Print and shaded views of the part. All mm, measured from the part's lowest x, y and z. A direction names the side the tool comes from. Coordinates: 2 decimals unless noted, no trailing zeros. Loops run counter-clockwise (first coordinate to the right, second up) from the corner with the lowest first, then second, coordinate; pieces in that order, holes last. Notation, with made-up numbers: M 35,-22 L 73,-22 A15 ccw 73,-18 Z; hole C -0.75,52.5 d8. An arc over 180 degrees is marked long. One line per question, with ' | ' between items. Start each with the question number.
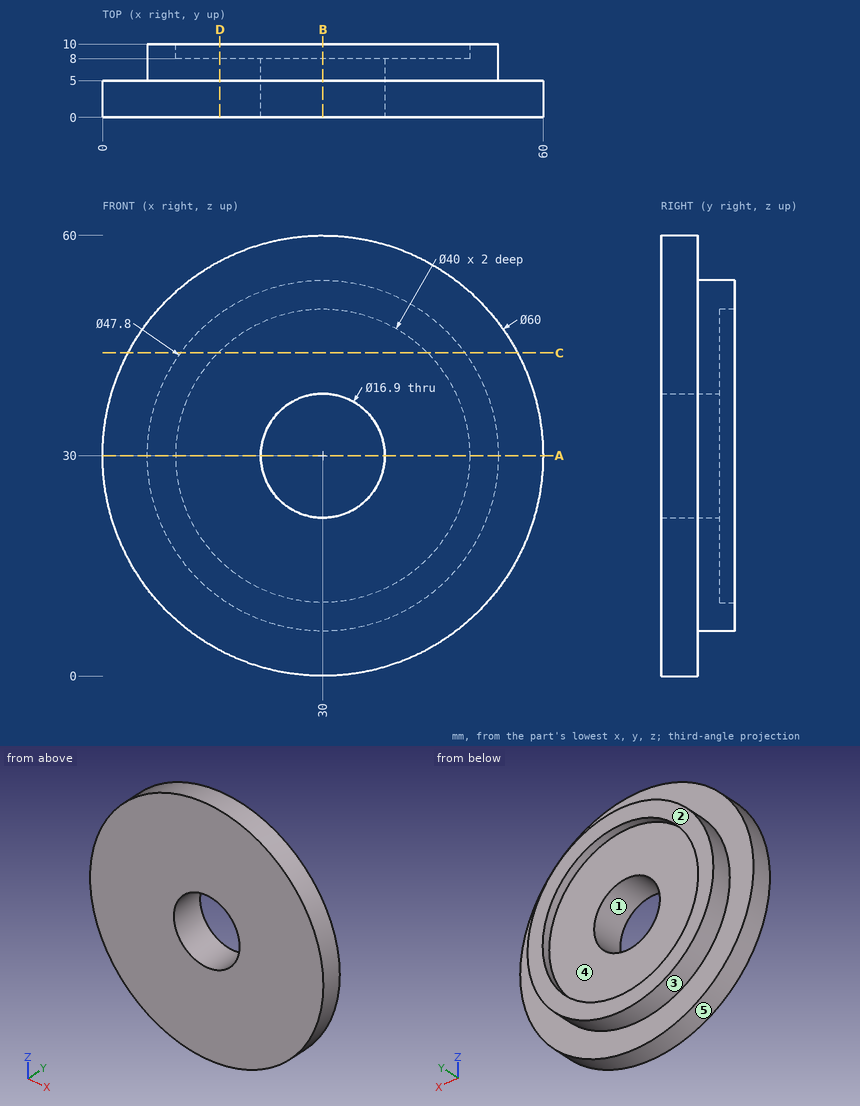
(1) Band-saw the part on B-B on x = 30. Write the cut outline in (y, z).
(2) Band-saw the part on C-C on z = 44. Write the cut outline in (x, y).
(3) Pin check, flat tips, straight feed: P1, Ø2, axis at x = 13, y = 5, coming from the +Z side; P2, Ø6, axis at x = 34.5, y = 2.5, coming from the +Z side; P3, Ø22, axis at x = 30, z = 30, coming from the +Y side. Stop position of each tip, or through.
(4) Drill centre lines: line 1 (X direction, y = 8.85, z = 30); line 2 (X direction, y = 4.5, z = 30). Where is each one in solid material? Low to high. Write a range as [from, to].
(5) Band-saw the part on D-D on x = 16. Write the cut outline in (y, z).
(6) Two-plate mould, pull along Z, no slides. Class the marked faces 1, 2 and 3: pulls with the +Z half, pulls with the -Z half, needs draft (parallel to the pull), parting line crosses it, or undercut.
(7) Band-saw the part on A-A on z = 30. Write the cut outline in (x, y).
(8) 3-axis set-ups, long thin cutter, end or side, ignore diameter. For the marked faces 4 and 5: which of +Z, -Z, +X, -X, +Y, -Y reach the whole face in a straight line?
Computed values:
1) outline: M 0,0 L 5,0 L 5,6.1 L 10,6.1 L 10,10 L 8,10 L 8,21.55 L 0,21.55 Z; M 0,38.45 L 8,38.45 L 8,50 L 10,50 L 10,53.9 L 5,53.9 L 5,60 L 0,60 Z
2) outline: M 3.47,0 L 56.53,0 L 56.53,5 L 49.37,5 L 49.37,10 L 44.28,10 L 44.28,8 L 15.72,8 L 15.72,10 L 10.63,10 L 10.63,5 L 3.47,5 Z
3) P1: z = 55.38 | P2: z = 59.96 | P3: y = 8
4) line 1: [6.1, 10], [50, 53.9] | line 2: [0, 21.55], [38.45, 60]
5) outline: M 0,3.47 L 5,3.47 L 5,10.63 L 10,10.63 L 10,15.72 L 8,15.72 L 8,44.28 L 10,44.28 L 10,49.37 L 5,49.37 L 5,56.53 L 0,56.53 Z
6) face 1: undercut | face 2: needs draft | face 3: parting line crosses it
7) outline: M 0,0 L 21.55,0 L 21.55,8 L 10,8 L 10,10 L 6.1,10 L 6.1,5 L 0,5 Z; M 38.45,0 L 60,0 L 60,5 L 53.9,5 L 53.9,10 L 50,10 L 50,8 L 38.45,8 Z
8) face 4: +Y | face 5: +Y, -Y
